Geometry: see drawing. Coordinates: mm, zero at the bounding-box minimum. Coordinates: 2 decimals unless noted, no trailing zeros. Loops run counter-clockwise (first coordinate to the right, second up) from the corner with the lowest first, then second, coordinate; pieces in that order, holes last.
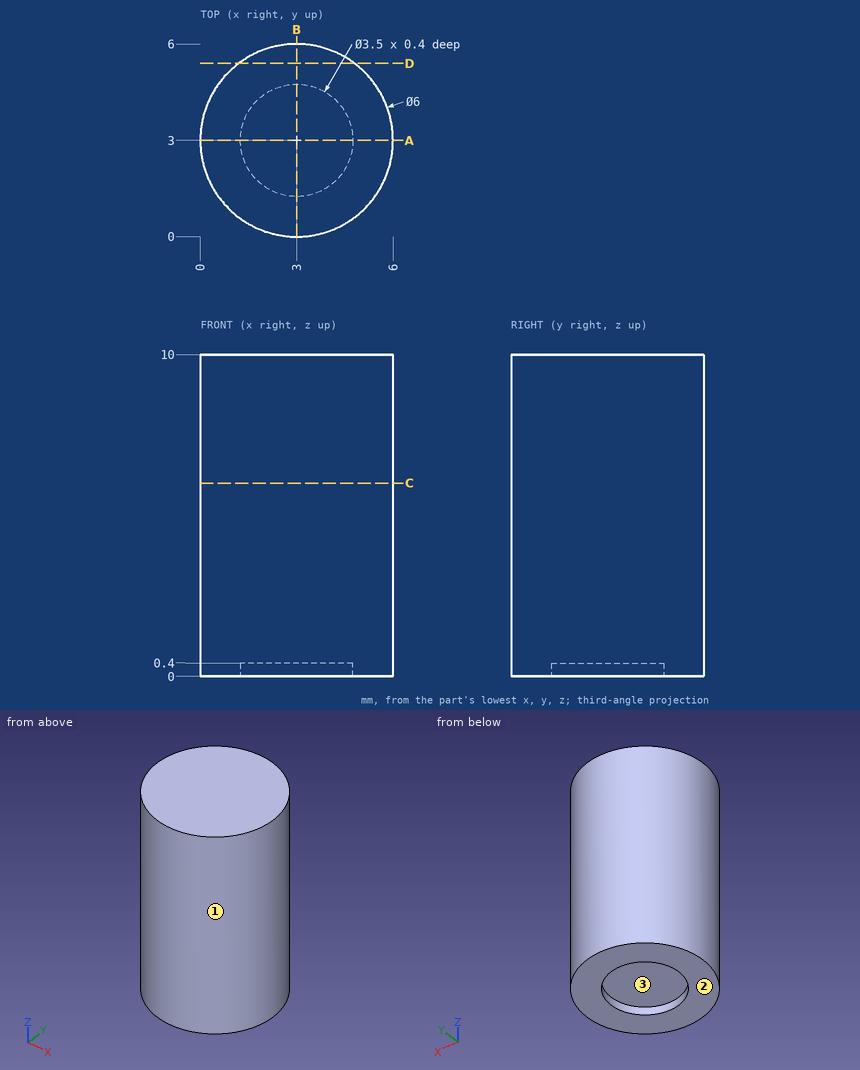
Item 1: Mould query, pull axis Y, two halves, no side actions, for the marked faces 1, 2 and 3. Classes: +Y half, -Y half, draft (parallel to the pull), parting line (faces both ways), or undercut.
Result:
face 1: parting line
face 2: draft
face 3: undercut
Item 2: Contact query for flat-ended pins moving along their axis: P1, Ø1.5, axis at y = 4, z = 5, coming from the +X side; P2, Ø2, axis at x = 2.5, y = 3.5, coming from the -Z side; P3, Ø1, axis at y = 5, z = 3, coming from the -X side. Output: stop coordinate, or through.
Result:
P1: stops at x = 5.99
P2: stops at z = 0.4
P3: stops at x = 0.4
Item 3: Line query: L1, parallel to Y at x = 3, z = 0.25; L2, parallel to Z at x = 2.85, y = 3.7; L3, parallel to Y at x = 3.1, z = 8.75. Output: solid intervals per line, ascending.
Result:
L1: y = 0 to 1.25, 4.75 to 6
L2: z = 0.4 to 10
L3: y = 0 to 6
Item 4: Section query C-C (z = 6). Output: boundary loops of the cut face in (x, y).
Result:
outline: circle Ø6 at (3, 3)
Item 5: Section query D-D (y = 5.4). Output: boundary loops of the cut face in (x, z).
Result:
outline: (1.2, 0) - (4.8, 0) - (4.8, 10) - (1.2, 10) - close
Item 6: Section query A-A (y = 3). Output: boundary loops of the cut face in (x, z).
Result:
outline: (0, 0) - (1.25, 0) - (1.25, 0.4) - (4.75, 0.4) - (4.75, 0) - (6, 0) - (6, 10) - (0, 10) - close
